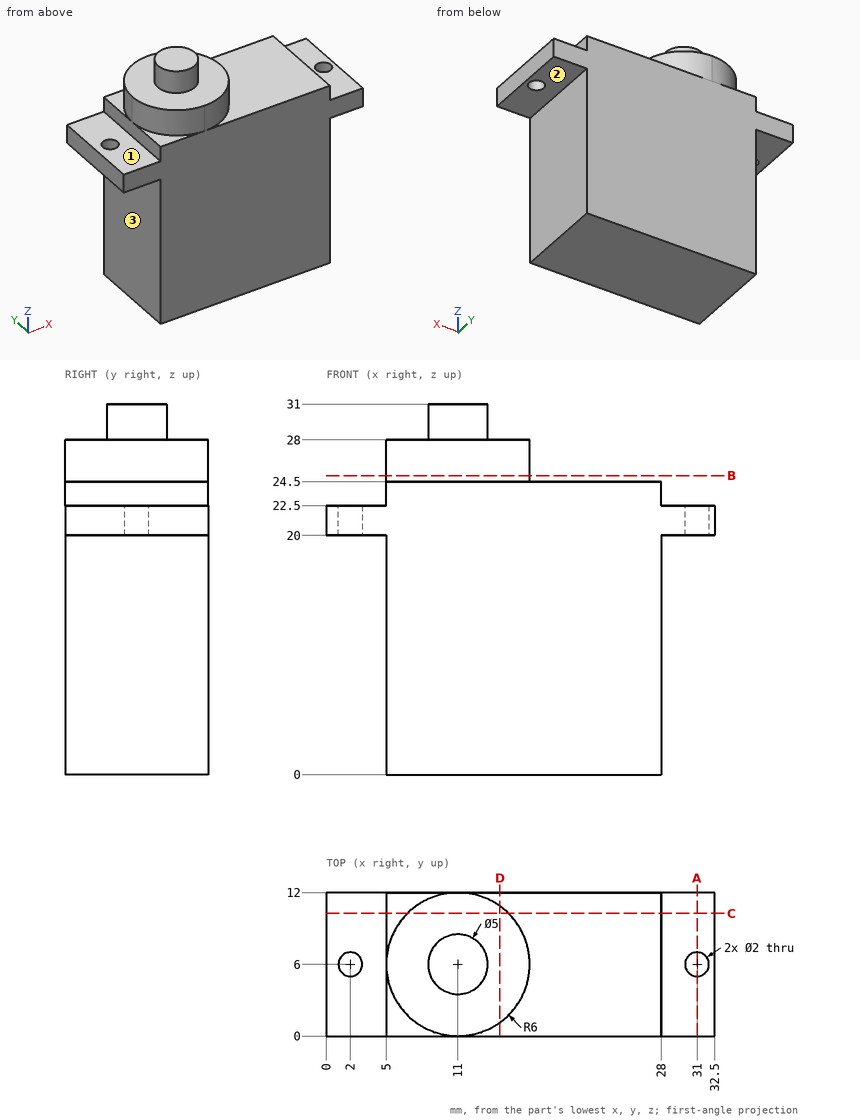
Here's the drawing with two shaded views (mm, measured from the low corner). I have some questions. A direction names the side the tool comes from. Coordinates: 2 decimals unless noted, no trailing zeros. Loops run counter-clockwise (first coordinate to the right, second up) from the corner with the lowest first, then second, coordinate; pieces in that order, holes last. Notation, with made-up numbers: (71, 56.5) - (85, 56.5) arc R20 cw to (85, 88.5) - close; hole circle Ø9 at (-14.75, 28). An arc over 180 degrees is marked (long way). Answer as CSV lines item,"result". Start each with the question number.
1) Suppose I cut it at C-C (y = 10.25). Please give me the cut outline in (x, z), plus the area to 3 significant figures.
2) Which directions (+Z, -Z, +X, -X, +Y, -Y) give clear straight access to the entire face, cutting with the end or side of a thin tool? Please do the marked faces 1, 2 and 3.
3) Suppose I cut it at A-A (x = 31). Please give me the cut outline in (y, z), plus the area to 3 significant figures.
4) I need wall thicknesses on line 1 (Y direction, x = 2, z = 21); line 2 (Z direction, x = 26, y = 9); line 3 (Z direction, x = 29, y = 4.75). Which ranges of each line are inside material? Lowest first, please. Write a range as from..to.
5) For pin 1 (3.5 mm diameter, centred on y = 5.5, z = 5.5, fed in from +X); pin 2 (5 mm diameter, centred on x = 30, y = 3.5, fed in from +Z); pin 3 (6 mm diameter, centred on x = 17.5, y = 4.5, fed in from +Z); pin 4 (1.6 mm diameter, centred on x = 31, y = 6, fed in from -Z), each with a flat end and sliding along its axis, tell me the tip position at first contact or that it passes through.
6) Suppose I cut it at D-D (x = 14.5). Please give me the cut outline in (y, z).
7) Suppose I cut it at B-B (z = 25). Please give me the cut outline in (x, y), plus the area to 3 significant figures.
Check result:
1,outline,"(0, 20) - (5, 20) - (5, 0) - (28, 0) - (28, 20) - (32.5, 20) - (32.5, 22.5) - (28, 22.5) - (28, 24.5) - (15.24, 24.5) - (15.24, 28) - (6.76, 28) - (6.76, 24.5) - (5, 24.5) - (5, 22.5) - (0, 22.5) - close"
1,area,"617 mm²"
2,face 1,"+Z, -X, +Y, -Y"
2,face 2,"-Z, +X, +Y, -Y"
2,face 3,"-Z, -X, +Y, -Y"
3,outline,"(0, 20) - (5, 20) - (5, 22.5) - (0, 22.5) - close; (7, 20) - (12, 20) - (12, 22.5) - (7, 22.5) - close"
3,area,"25.0 mm²"
4,line 1,"y = 0..5, 7..12"
4,line 2,"z = 0..24.5"
4,line 3,"z = 20..22.5"
5,pin 1,"stops at x = 28"
5,pin 2,"stops at z = 24.5"
5,pin 3,"stops at z = 28"
5,pin 4,"passes through"
6,outline,"(0, 0) - (12, 0) - (12, 24.5) - (10.87, 24.5) - (10.87, 28) - (1.13, 28) - (1.13, 24.5) - (0, 24.5) - close"
7,outline,"circle Ø12 at (11, 6)"
7,area,"113 mm²"
